CAD build for the part. Positions are in the model's coordinates, mm. Face numbers are marked on the shaded views. A direction names the side the tool comes from. Round coordinates to 2 decimals unless told otherwise and drop trailing zeros. Use one line per item in the form item = value. Start each with the question number.
Item 1: Tool access for the marked faces 1, 2, 3 and 4: list every direction of +Z, -Z, +X, -X, +Y, -Y with a clear straight run to the whole face (end or side of a thin tool).
Item 2: Pin check, flat tips, straight feed: pin 1 (5.5 mm diameter, centred on x = -35.5, y = -2.5, fed in from -Z); pin 2 (5.5 mm diameter, centred on x = -35.5, y = -37, fed in from -Z); pin 3 (5.5 mm diameter, centred on x = 6.5, z = 1.5, fed in from -Y). Stop position of each tip, or through.
Item 3: Pull direction X, two halves, no side cores. Call the marked faces 5, 6 and 7: +X half, -X half, draft (parallel to the pull), parting line (faces both ways), or undercut.
Item 4: Drill centre lines: L1, parallel to X at y = -48.5, z = 26; L2, parallel to Y at x = -23.5, z = 34.5; L3, parallel to Z at x = -44, y = 18. Where is each one in solid material? Low to high.
Item 5: Band-saw the part on A-A, the plane x = -13. Give the number of separate pieces and of enclosed holes in the cut face, and give its area (3 significant figures).
from build123d import *

# Parameters (mm, degrees)
SKETCH_1_W           = 74
SKETCH_1_H           = 120
EXTRUDE_1_DEPTH      = 70
CHAMFER_2_SIZE       = 30
SHELL_1_T            = -5
CUT_EXTRUDE_1_DEPTH  = 119.220133649
SKETCH_3_W           = 54
SKETCH_3_H           = 22.426406871
CUT_EXTRUDE_2_DEPTH  = 70
SKETCH_4_W           = 54
SKETCH_4_H           = 22.426406871
CUT_EXTRUDE_3_DEPTH  = 70
SKETCH_5_W           = 54
SKETCH_5_H           = 40
CUT_EXTRUDE_4_DEPTH  = 70
SKETCH_7_W           = 54
SKETCH_7_H           = 20
CUT_EXTRUDE_5_DEPTH  = 144.767172887
FILLET_1_R           = 5
EXTRUDE_3_DEPTH      = 15
EXTRUDE_3_DEPTH_BACK = 5
SKETCH_10_W          = 70
SKETCH_10_H          = 5
SKETCH_12_R          = 2.1
CUT_EXTRUDE_7_DEPTH  = 119.33849754
SKETCH_13_R          = 1.6
CUT_EXTRUDE_8_DEPTH  = 10


with BuildPart() as part:
    # ｽｹｯﾁ1 → ﾎﾞｽ - 押し出し1 (new body)
    with BuildSketch(Plane.XY):
        Rectangle(SKETCH_1_W, SKETCH_1_H)
    extrude(amount=EXTRUDE_1_DEPTH)

    # 面取り2
    chamfer_2_edges = [part.edges().sort_by_distance(p)[0] for p in [
        (0, -60, 0),
        (0, 60, 0),
    ]]
    chamfer(chamfer_2_edges, length=CHAMFER_2_SIZE)

    # ｼｪﾙ1
    shell_1_openings = [part.faces().sort_by_distance(p)[0] for p in [
        (0, 0, 70),
    ]]
    offset(amount=SHELL_1_T, openings=shell_1_openings, kind=Kind.INTERSECTION)

    # ｽｹｯﾁ2 → ｶｯﾄ - 押し出し1 (cut, through all)
    with BuildSketch(Plane.ZY.offset(37)):
        Polygon((34.142135624, -50), (50, -50), (50, -26.558112383), (34.5, -17.60918321), (13.738168081, -29.596032457), align=None)
        Polygon((10, 20.207259422), (10, -20.207259422), (29.5, -8.948929172), (29.5, 8.948929172), align=None)
        Polygon((34.142135624, 50), (13.738168081, 29.596032457), (34.5, 17.60918321), (50, 26.558112383), (50, 50), align=None)
        with BuildLine():
            ThreePointArc((60, 9.233092656), (44.5, 0), (60, -9.233092656))
            Line((60, -9.233092656), (60, 9.233092656))
        make_face()
        with BuildLine():
            Line((60, 9.233092656), (60, -9.233092656))
            ThreePointArc((60, -9.233092656), (64.020809276, -5.373546315), (65.5, 0))
            ThreePointArc((65.5, 0), (64.020809276, 5.373546315), (60, 9.233092656))
        make_face()
    extrude(amount=-CUT_EXTRUDE_1_DEPTH, mode=Mode.SUBTRACT)

    # ｽｹｯﾁ3 → ｶｯﾄ - 押し出し2 (cut)
    with BuildSketch(Plane(origin=(0, -15, -15), x_dir=(1, 0, 0), z_dir=(0, -0.7071067811865464, -0.7071067811865487))):
        with Locations((0, 42.426406872)):
            Rectangle(SKETCH_3_W, SKETCH_3_H)
    extrude(amount=-CUT_EXTRUDE_2_DEPTH, mode=Mode.SUBTRACT)

    # ｽｹｯﾁ4 → ｶｯﾄ - 押し出し3 (cut)
    with BuildSketch(Plane(origin=(0, 15, -15), x_dir=(1, 0, 0), z_dir=(0, 0.7071067811865464, -0.7071067811865487))):
        with Locations((0, -42.426406872)):
            Rectangle(SKETCH_4_W, SKETCH_4_H)
    extrude(amount=-CUT_EXTRUDE_3_DEPTH, mode=Mode.SUBTRACT)

    # ｽｹｯﾁ5 → ｶｯﾄ - 押し出し4 (cut)
    with BuildSketch(Plane(origin=(0, 0, 0), x_dir=(-1, 0, 0), z_dir=(0, 0, -1))):
        Rectangle(SKETCH_5_W, SKETCH_5_H)
    extrude(amount=-CUT_EXTRUDE_4_DEPTH, mode=Mode.SUBTRACT)

    # ｽｹｯﾁ7 → ｶｯﾄ - 押し出し5 (cut, through all)
    with BuildSketch(Plane(origin=(0, 60, 0), x_dir=(1, 0, 0), z_dir=(0, 1, 0))):
        with Locations((0, -50)):
            Rectangle(SKETCH_7_W, SKETCH_7_H)
    extrude(amount=-CUT_EXTRUDE_5_DEPTH, mode=Mode.SUBTRACT)

    # ﾌｨﾚｯﾄ1
    fillet_1_edges = [part.edges().sort_by_distance(p)[0] for p in [
        (34.5, 20.207259422, 10),
        (34.5, 8.948929172, 29.5),
        (34.5, -8.948929172, 29.5),
        (34.5, -20.207259422, 10),
        (-34.5, 20.207259422, 10),
        (-34.5, 8.948929172, 29.5),
        (-34.5, -8.948929172, 29.5),
        (-34.5, -20.207259422, 10),
        (0, 60, 30),
        (-27, -51.161165235, 24.696699141),
        (27, -51.161165235, 24.696699141),
        (27, -35.303300859, 8.838834765),
        (-27, -35.303300859, 8.838834765),
        (-37, 0, 0),
        (-37, -45, 15),
        (-37, 45, 15),
        (27, 51.161165235, 24.696699141),
        (-27, 51.161165235, 24.696699141),
        (-27, 35.303300859, 8.838834765),
        (27, 35.303300859, 8.838834765),
        (37, 0, 0),
        (0, -30, 0),
        (0, 30, 0),
        (37, -45, 15),
        (-27, -20, 2.5),
        (27, -20, 2.5),
        (27, 20, 2.5),
        (-27, 20, 2.5),
        (37, 45, 15),
        (0, -60, 30),
        (27, 57.5, 60),
        (-27, 57.5, 60),
        (-27, 57.5, 40),
        (27, 57.5, 40),
        (27, -57.5, 60),
        (-27, -57.5, 60),
        (-27, -57.5, 40),
        (27, -57.5, 40),
        (34.5, -50, 34.142135624),
        (34.5, -29.596032457, 13.738168081),
        (34.5, -17.60918321, 34.5),
        (34.5, -26.558112383, 50),
        (34.5, -50, 50),
        (-34.5, -50, 34.142135624),
        (-34.5, -29.596032457, 13.738168081),
        (-34.5, -17.60918321, 34.5),
        (-34.5, -26.558112383, 50),
        (-34.5, -50, 50),
        (37, -60, 50),
        (-37, -60, 50),
        (-37, 60, 50),
        (37, 60, 50),
        (34.5, 50, 34.142135624),
        (34.5, 50, 50),
        (34.5, 26.558112383, 50),
        (34.5, 17.60918321, 34.5),
        (34.5, 29.596032457, 13.738168081),
        (-34.5, 50, 34.142135624),
        (-34.5, 50, 50),
        (-34.5, 26.558112383, 50),
        (-34.5, 17.60918321, 34.5),
        (-34.5, 29.596032457, 13.738168081),
    ]]
    fillet(fillet_1_edges, radius=FILLET_1_R)

    # ｽｹｯﾁ10 → ﾎﾞｽ - 押し出し3 (add, two sides: drawn at the far end of the back side and taken through both)
    with BuildSketch(Plane.ZY.offset(37).offset(-EXTRUDE_3_DEPTH_BACK)):
        with Locations((35, 17.5)):
            Rectangle(SKETCH_10_W, SKETCH_10_H)
        with Locations((35, -17.5)):
            Rectangle(SKETCH_10_W, SKETCH_10_H)
    extrude(amount=EXTRUDE_3_DEPTH + EXTRUDE_3_DEPTH_BACK)

    # ｽｹｯﾁ12 → ｶｯﾄ - 押し出し7 (cut, through all)
    with BuildSketch(Plane.XZ.offset(20)):
        with Locations((-44.5, 62.5)):
            Circle(SKETCH_12_R)
        with Locations((-44.5, 12.5)):
            Circle(SKETCH_12_R)
    extrude(amount=-CUT_EXTRUDE_7_DEPTH, mode=Mode.SUBTRACT)

    # ｽｹｯﾁ13 → ｶｯﾄ - 押し出し8 (cut)
    with BuildSketch(Plane(origin=(37, 0, 0), x_dir=(0, 0, -1), z_dir=(1, 0, 0))):
        with Locations(Location((-12.349364905, 24.624355653, 0), (0, 0, 90))):
            Circle(SKETCH_13_R)
        with Locations(Location((-34, 12.124355653, 0), (0, 0, 90))):
            Circle(SKETCH_13_R)
        with Locations(Location((-34, -10.011106999, 0), (0, 0, 90))):
            Circle(SKETCH_13_R)
        with Locations(Location((-12.349364905, -22.511106999, 0), (0, 0, 90))):
            Circle(SKETCH_13_R)
    extrude(amount=-CUT_EXTRUDE_8_DEPTH, mode=Mode.SUBTRACT)


solid = part.part
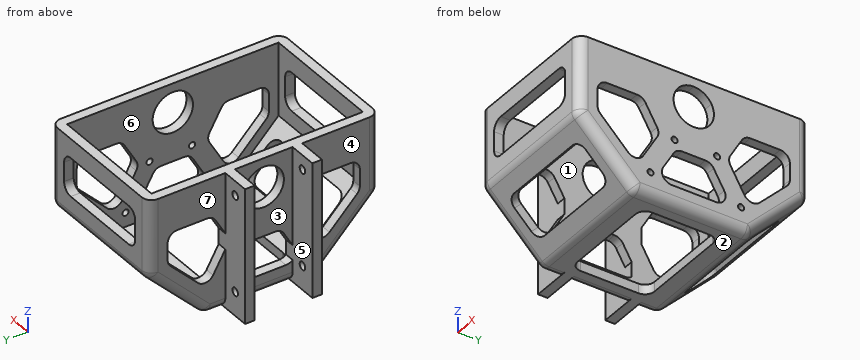
Determined:
q1.face_1 = +Z
q1.face_2 = -Z, +X, -X, +Y, -Y
q1.face_3 = +Z, -Z, -X
q1.face_4 = +Z, -Z, -X, -Y
q2.pin_1 = 0.06
q2.pin_2 = 5.28
q2.pin_3 = -34.25
q3.face_5 = draft
q3.face_6 = undercut
q3.face_7 = -X half
q4.L1 = -37 to -32, 32 to 37
q4.L2 = -60 to -55, 55 to 60
q4.L3 = 0 to 10.46, 14.54 to 60.46, 64.54 to 70
q5.separate_pieces = 6
q5.enclosed_holes = 0
q5.area = 456 mm²
